Can you work these out from the model? Positions are in its coordinate system, mm. A direction names the side the tool comes from. Coordinates: 2 decimals unless noted, no trailing zeros. Order: outer loops, then holes, each group sorted by start corner. A loop starts at its lowest first (then second) coordinate and runs counter-clockwise, first axis right, second up. Notation, with made-up numbers: (3.25, 21) -> (26.25, 21) arc R23 cw to (26.25, 35) -> close; hole circle Ø5 at (31.5, 81). An arc over 180 degrees is marked (long way). Use a Markdown table: item, result. Add a question column.
1. For faces 1 (the flat face through (-58, -26, 20.638)), 2 (the flat face through (-29, -15, 50.8)), 3 (the flat face through (-91, -50.787, 19)), which set-ups out of +Z, -Z, +X, -X, +Y, -Y let a thin tool reach every point of the face, with its end or its side?
2. We'd pull the mould along X, two halves only. Please class faces 4 (the flat face through (-55.789, -26, 25)), 5 (the cylindrical face through (25.394, -14.87, 24.841)), 6 (the flat face through (-29, -15, 0)): pulls with the +X half, pulls with the -X half, needs draft (parallel to the pull), parting line crosses it, or undercut.
3. Suppose I cut it at B-B, the plane x = -86.5. List the corners of the cut face in (y, z) for me.
4. For pin 1 Ø1 at (x, y) = (-91, -6) entering from +Z; pin 2 Ø4 at (x, y) = (-57.5, -13) entering from +Z; pin 3 Ø1.5 at (x, y) = (-5, -7) entering from +Z, each with a flat end and sliding along its axis, tell me the tip position at first contact or that it passes through.
5. Suppose I cut it at C-C, the plane y = -25.5. State how many separate pieces and enclosed holes the cut face has, then the cut area to 3 significant figures.
6. Suppose I cut it at D-D, the plane x = 5. List the corners of the cut face in (y, z) for me.
7. If I drill on line 1 along X through (y, z) = (-20, 25); line 2 along Z through (x, y) = (-76, -14); line 3 along X through (y, z) = (-31, 25), over which ranges is the centre line in solid material (lowest first)? Write a range as from..to.
```python
from build123d import *

# Parameters (mm, degrees)
F0_W     = 76.2
F0_H     = 50.8
F1_DEPTH = 30.1625
F3_DEPTH = 30.1752
F4_DEPTH = 20.6248
F5_DEPTH = 20.6248
F7_DEPTH = 50.8
F8_R     = 9.525
F9_DEPTH = 30.1752


with BuildPart() as f1:
    # F0 (on Front) → F1 (new body)
    with BuildSketch(Plane.XZ):
        with Locations((-38.1, 25.4)):
            Rectangle(F0_W, F0_H)
        with BuildLine():
            Line((0, 50.8), (0, 0))
            ThreePointArc((0, 0), (25.4, 25.4), (0, 50.8))
        make_face()
    extrude(amount=F1_DEPTH)

    # F2 (on face) → F3 (join)
    with BuildSketch(Plane.XZ.offset(30.1625)):
        with BuildLine():
            Line((-76.2, 50.8), (-57.15, 50.8))
            ThreePointArc((-57.15, 50.8), (-107.95, 25.4), (-57.15, 0))
            Line((-57.15, 0), (-76.2, 0))
            Line((-76.2, 0), (-76.2, 50.8))
        make_face()
    extrude(amount=-F3_DEPTH)

    # F2 (on face) → F4 (join)
    with BuildSketch(Plane.XZ.offset(30.1625)):
        with BuildLine():
            Line((-76.2, 50.8), (-57.15, 50.8))
            ThreePointArc((-57.15, 50.8), (-107.95, 25.4), (-57.15, 0))
            Line((-57.15, 0), (-76.2, 0))
            Line((-76.2, 0), (-76.2, 50.8))
        make_face()
    extrude(amount=F4_DEPTH)

    # F2 (on face) → F5 (join)
    with BuildSketch(Plane.XZ.offset(30.1625)):
        with BuildLine():
            ThreePointArc((-57.15, 0), (-47.8019366858, 11.2009683429), (-44.45, 25.4))
            ThreePointArc((-44.45, 25.4), (-47.8019366858, 39.5990316571), (-57.15, 50.8))
            Line((-57.15, 50.8), (-76.2, 50.8))
            Line((-76.2, 50.8), (-76.2, 0))
            Line((-76.2, 0), (-57.15, 0))
        make_face()
        with BuildLine():
            Line((-76.2, 50.8), (-57.15, 50.8))
            ThreePointArc((-57.15, 50.8), (-107.95, 25.4), (-57.15, 0))
            Line((-57.15, 0), (-76.2, 0))
            Line((-76.2, 0), (-76.2, 50.8))
        make_face()
    extrude(amount=F5_DEPTH)

    # F6 (on face) → F7 (cut)
    with BuildSketch(Plane.XZ.offset(50.7873)):
        with BuildLine():
            Line((-76.2, 25.4), (-60.325, 25.4))
            ThreePointArc((-60.325, 25.4), (-60.5088686027, 27.8091534761), (-61.0562151775, 30.1625))
            ThreePointArc((-61.0562151775, 30.1625), (-66.8082233443, 38.1988341754), (-76.2, 41.275))
            Line((-76.2, 41.275), (-76.2, 25.4))
        make_face()
        with BuildLine():
            Line((-55.7891130447, 25.4), (-60.325, 25.4))
            ThreePointArc((-60.325, 25.4), (-60.5088686027, 22.9908465239), (-61.0562151775, 20.6375))
            Line((-61.0562151775, 20.6375), (-55.7891130447, 20.6375))
            Line((-55.7891130447, 20.6375), (-55.7891130447, 25.4))
        make_face()
        with BuildLine():
            ThreePointArc((-61.0562151775, 20.6375), (-60.5088686027, 22.9908465239), (-60.325, 25.4))
            Line((-60.325, 25.4), (-76.2, 25.4))
            Line((-76.2, 25.4), (-76.2, 9.525))
            ThreePointArc((-76.2, 9.525), (-66.8082233443, 12.6011658246), (-61.0562151775, 20.6375))
        make_face()
        with BuildLine():
            ThreePointArc((-61.0562151775, 30.1625), (-60.5088686027, 27.8091534761), (-60.325, 25.4))
            Line((-60.325, 25.4), (-55.7891130447, 25.4))
            Line((-55.7891130447, 25.4), (-55.7891130447, 30.1625))
            Line((-55.7891130447, 30.1625), (-61.0562151775, 30.1625))
        make_face()
        with BuildLine():
            Line((-76.2, 9.525), (-76.2, 25.4))
            Line((-76.2, 25.4), (-76.2, 41.275))
            ThreePointArc((-76.2, 41.275), (-92.075, 25.4), (-76.2, 9.525))
        make_face()
    extrude(amount=-F7_DEPTH, mode=Mode.SUBTRACT)

    # F8 (on face) → F9 (cut)
    with BuildSketch(Plane.XZ.offset(30.1625)):
        with Locations((0, 25.4230257124)):
            Circle(F8_R)
    extrude(amount=-F9_DEPTH, mode=Mode.SUBTRACT)


solid = f1.part
```
Worked out:
| question | item | result |
|---|---|---|
| 1 | face 1 | +Y, -Y |
| 1 | face 2 | +Z, +X, +Y, -Y |
| 1 | face 3 | +Z, -Z, +X, -X, -Y |
| 2 | face 4 | undercut |
| 2 | face 5 | pulls with the +X half |
| 2 | face 6 | needs draft |
| 3 | outline | (-50.79, -4.63) -> (0.01, -4.63) -> (0.01, 13.32) -> (-50.79, 13.32) -> close; (-50.79, 37.48) -> (0.01, 37.48) -> (0.01, 55.43) -> (-50.79, 55.43) -> close |
| 4 | pin 1 | stops at z = 53.75 |
| 4 | pin 2 | stops at z = 52.4 |
| 4 | pin 3 | stops at z = 50.8 |
| 5 | separate pieces | 1 |
| 5 | enclosed holes | 2 |
| 5 | area | 5,510 mm² |
| 6 | outline | (-30.16, 0.5) -> (0, 0.5) -> (0, 17.32) -> (-30.16, 17.32) -> close; (-30.16, 33.53) -> (0, 33.53) -> (0, 50.3) -> (-30.16, 50.3) -> close |
| 7 | line 1 | x = -107.95..-92.07, -55.79..-9.52, 9.52..25.4 |
| 7 | line 2 | z = -6.35..9.53, 41.27..57.15 |
| 7 | line 3 | x = -107.95..-92.07, -55.79..-44.45 |
